Part model, mm, in its own coordinate system. A direction names the side the tool comes from. Round coordinates to 2 decimals unless told otherwise and drop trailing zeros. Write each loop counter-clockwise with the first axis right and the second up, starting at its lowest first coordinate (ties: lowest second). Pieces come first, ordered by that corner, then holes.
```python
from build123d import *

# Parameters (mm, degrees)
F0_W      = 25
F0_H      = 25
F1_DEPTH  = 30
F3_DEPTH  = 25.001
F4_R      = 2.1
F5_DEPTH  = 25.001
F6_R      = 5
F7_DEPTH  = 22
F9_DEPTH  = 7
F10_R     = 2.6
F11_DEPTH = 15
F14_W     = 30
F14_H     = 12.5
F15_DEPTH = 25
F16_DEPTH = 7
F18_DEPTH = 10
F20_DEPTH = 10
F22_D     = 8
F24_DEPTH = 12.5
F25_W     = 9.5
F25_H     = 25
F26_DEPTH = 3
F28_D     = 4.2
F28_DEPTH = 15
F28_TIP   = 1.2618073
F31_D     = 2.5
F31_DEPTH = 8
F31_TIP   = 0.7510757738


with BuildPart() as f1:
    # F0 (on Right) → F1 (new body, symmetric)
    with BuildSketch(Plane.YZ):
        Rectangle(F0_W, F0_H)
    extrude(amount=F1_DEPTH, both=True)

    # F2 (on face) → F3 (cut, through all)
    with BuildSketch(Plane.XY.offset(12.5)):
        with BuildLine():
            Line((12, -12.5), (22, -12.5))
            ThreePointArc((22, -12.5), (17, -7.5), (12, -12.5))
        make_face()
    extrude(amount=-F3_DEPTH, mode=Mode.SUBTRACT)

    # F4 (on face) → F5 (cut, through all)
    with BuildSketch(Plane.XY.offset(12.5)):
        with Locations((17, -4.5)):
            Circle(F4_R)
    extrude(amount=-F5_DEPTH, mode=Mode.SUBTRACT)

    # F6 (on face) → F7 (cut)
    with BuildSketch(Plane(origin=(0, 0, -12.5), x_dir=(1, 0, 0), z_dir=(0, 0, -1))):
        with Locations((5, 5.5)):
            Circle(F6_R)
    extrude(amount=-F7_DEPTH, mode=Mode.SUBTRACT)

    # F8 (on face) → F9 (cut)
    with BuildSketch(Plane.XZ.offset(12.5)):
        with BuildLine():
            Line((1.5, -12.5), (8.5, -12.5))
            Line((8.5, -12.5), (8.5, 2.5))
            ThreePointArc((8.5, 2.5), (5, 6), (1.5, 2.5))
            Line((1.5, 2.5), (1.5, -12.5))
        make_face()
    extrude(amount=-F9_DEPTH, mode=Mode.SUBTRACT)

    # F10 (on face) → F11 (cut)
    with BuildSketch(Plane(origin=(0, 0, -12.5), x_dir=(1, 0, 0), z_dir=(0, 0, -1))):
        with Locations((17, 4.5)):
            Circle(F10_R)
    extrude(amount=-F11_DEPTH, mode=Mode.SUBTRACT)


with BuildPart() as f12_1:
    # F12: copy of F1
    add(f1.part)


with BuildPart() as f1_1:
    add(f1.part)

    # F14 (on face) → F15 (join)
    with BuildSketch(Plane(origin=(0, 0, -12.5), x_dir=(1, 0, 0), z_dir=(0, 0, -1))):
        with Locations((15, -6.25)):
            Rectangle(F14_W, F14_H)
    extrude(amount=F15_DEPTH)

    # F16 (add): a face of the model
    f16_faces = [f1_1.faces().sort_by_distance(p)[0] for p in [
        (5, 12.5, -8.3333333333),
    ]]
    extrude(f16_faces, amount=F16_DEPTH)

    # F17 (on face) → F18 (cut)
    with BuildSketch(Plane(origin=(0, 19.5, 0), x_dir=(-1, 0, 0), z_dir=(0, 1, 0))):
        Polygon((-30, -5), (-6.4768494526, 0), (30, 0), (30, 12.5), (-30, 12.5), align=None)
    extrude(amount=-F18_DEPTH, mode=Mode.SUBTRACT)

    # F19 (on face) → F20 (cut)
    with BuildSketch(Plane(origin=(0, 19.5, 0), x_dir=(-1, 0, 0), z_dir=(0, 1, 0))):
        Polygon((30, -1.2575895653), (-12.3933431868, -1.2575895653), (-4.6897810382, -37.5), (0, -37.5), (0, -12.5), (30, -12.5), align=None)
        Polygon((-12.3933431868, 5.6717685307), (-12.3933431868, -1.2575895653), (-6.4768494526, 0), (30, 0), (30, 5.6717685307), align=None)
        Polygon((-6.4768494526, 0), (-12.3933431868, -1.2575895653), (30, -1.2575895653), (30, 0), align=None)
    extrude(amount=-F20_DEPTH, mode=Mode.SUBTRACT)

    # F22 (through all)
    with Locations(Plane(origin=(0.2799765277, 0, 1.317186002), x_dir=(0.9781476007, 0, -0.2079116908), z_dir=(0.2079116908, 0, 0.9781476007))):
        with Locations((27.3839864761, 14.5)):
            Hole(F22_D / 2)

    # F23 (on face) → F24 (cut)
    with BuildSketch(Plane.XY.offset(12.5)):
        Polygon((21.3397459622, 2.5), (30, -12.5), (30, 9.5), (17.2982940778, 9.5), align=None)
        Polygon((-30, 2.5), (21.3397459622, 2.5), (17.2982940778, 9.5), (-30, 9.5), align=None)
    extrude(amount=-F24_DEPTH, mode=Mode.SUBTRACT)

    # F25 (on face) → F26 (cut)
    with BuildSketch(Plane.YZ.offset(30)):
        with BuildLine():
            Line((-12.5, 0), (-12.5, -12.5))
            Line((-12.5, -12.5), (0, -12.5))
            Line((0, -12.5), (9.5, -12.5))
            Line((9.5, -12.5), (19.5, -12.5))
            Line((19.5, -12.5), (19.5, -5))
            Line((19.5, -5), (17.1457513111, -5))
            add(Edge.make_bspline(
                [(14.5, -9.8097343447), (16.011857892, -9.8097343447), (17.1457513111, -5)],
                knots=[3.1415926536, 3.1415926536, 3.1415926536, 3.8643269014, 3.8643269014, 3.8643269014], degree=2, weights=[1, 0.9354143467, 1]))
            add(Edge.make_bspline(
                [(11.8542486889, -5), (12.988142108, -9.8097343447), (14.5, -9.8097343447)],
                knots=[2.4188584058, 2.4188584058, 2.4188584058, 3.1415926536, 3.1415926536, 3.1415926536], degree=2, weights=[1, 0.9354143467, 1]))
            Line((11.8542486889, -5), (9.5, -5))
            Line((9.5, -5), (9.5, 0))
            Line((9.5, 0), (-12.5, 0))
        make_face()
        with BuildLine():
            Line((-12.5, 12.5), (-12.5, 0))
            Line((-12.5, 0), (9.5, 0))
            Line((9.5, 0), (9.5, -5))
            Line((9.5, -5), (11.8542486889, -5))
            add(Edge.make_bspline(
                [(11.8542486889, -5), (12.988142108, -9.8097343447), (14.5, -9.8097343447)],
                knots=[2.4188584058, 2.4188584058, 2.4188584058, 3.1415926536, 3.1415926536, 3.1415926536], degree=2, weights=[1, 0.9354143467, 1]))
            add(Edge.make_bspline(
                [(14.5, -9.8097343447), (16.011857892, -9.8097343447), (17.1457513111, -5)],
                knots=[3.1415926536, 3.1415926536, 3.1415926536, 3.8643269014, 3.8643269014, 3.8643269014], degree=2, weights=[1, 0.9354143467, 1]))
            Line((17.1457513111, -5), (19.5, -5))
            Line((19.5, -5), (19.5, 12.5))
            Line((19.5, 12.5), (-12.5, 12.5))
        make_face()
        with Locations((4.75, -25)):
            Rectangle(F25_W, F25_H)
    extrude(amount=-F26_DEPTH, mode=Mode.SUBTRACT)

    # F28
    with Locations(Plane(origin=(12.1133666591, 0, -2.5747755673), x_dir=(0, -1, 0), z_dir=(-0.9781476007, 0, 0.2079116908))):
        with Locations((-14.5, -7.7054747223), (-14.5, -17.7054747223), (-14.5, -27.7054747223)):
            Hole(F28_D / 2, depth=F28_DEPTH)
            with Locations((0, 0, -(F28_DEPTH + F28_TIP / 2))):  # 118° drill point
                Cone(0, F28_D / 2, F28_TIP, mode=Mode.SUBTRACT)

    # F31
    with Locations(Plane(origin=(17.0873412263, 9.8653810568, 0), x_dir=(-0.5, 0.8660254038, 0), z_dir=(0.8660254038, 0.5, 0))):
        with Locations((-12.397114317, 9.5)):
            Hole(F31_D / 2, depth=F31_DEPTH)
            with Locations((0, 0, -(F31_DEPTH + F31_TIP / 2))):  # 118° drill point
                Cone(0, F31_D / 2, F31_TIP, mode=Mode.SUBTRACT)


solid = f1_1.part
```
Q1. Cut at B-B on y = -5.5. Write the cut outline in (x, z).
Values follow:
outline: (-30, -12.5) - (0, -12.5) - (0, 9.5) - (10, 9.5) - (10, -12.5) - (14.6, -12.5) - (14.6, 2.5) - (15.15, 2.5) - (15.15, 12.5) - (-30, 12.5) - close; (18.85, 2.5) - (19.4, 2.5) - (19.4, -12.5) - (27, -12.5) - (27, 0) - (25.96, 0) - (25.96, 12.5) - (18.85, 12.5) - close
Q2. Cut at C-C on x = -21. Write the cut outline in (y, z).
Values follow:
outline: (-12.5, -12.5) - (9.5, -12.5) - (9.5, 0) - (2.5, 0) - (2.5, 12.5) - (-12.5, 12.5) - close
Q3. Which spindle directions (+Z, -Z, +X, -X, +Y, -Y) get a long thin tool onto all of the face, cutting with end or side? Do faces 4 (the flat face through (24.13, -2.33, 6.34)), 5 (the cylindrical face through (15.334, -5.778, 7.57)), 6 (the flat face through (29.5, 13.3, -12.5)), 7 (the flat face through (-9, -12.5, 0)), 8 (the cylindrical face through (19.48, -5.28, -5.11)). Say none if no direction does.
Values follow:
face 4: +Z, +X, +Y
face 5: +Z, -Z
face 6: +Z, +X, +Y, -Y
face 7: +Z, -Z, +X, -X, -Y
face 8: -Z
Q4. Mould opens along Z. For faces 1 (the flat face through (27, 19, -8)), 2 (the cylindrical face through (5, -11, 6)), 3 (the cylindrical face through (12.235, 16.503, -30.28)) say: +Z half, -Z half, draft (parallel to the pull), parting line (faces both ways), or undercut.
Values follow:
face 1: draft
face 2: -Z half
face 3: undercut
Q5. Wall check: L1, parallel to Y at x = 17, z = 8; L2, parallel to X at y = -5.5, z = -3; L3, parallel to Z at x = 9, y = 8. Give the ranges that are in metal, low to high.
Values follow:
L1: y = -7.5 to -6.6, -2.4 to 2.5
L2: x = -30 to 0, 10 to 14.6, 19.4 to 27
L3: z = -37.5 to 0
Q6. Cut at A-A on z = 1.5. Write the cut outline in (x, y), plus the area to 3 significant figures.
Values follow:
outline: (-30, -12.5) - (1.5, -12.5) - (1.5, -9.07) arc R5 cw (long way) to (8.5, -9.07) - (8.5, -12.5) - (12, -12.5) arc R5 cw to (22, -12.5) - (27, -12.5) - (27, -7.3) - (21.34, 2.5) - (-30, 2.5) - close; hole circle Ø5.2 at (17, -4.5)
area: 671 mm2
Q7. Drop flat-ended pins along their axis: pin 1 (8 mm diameter, centred on x = -7.5, y = -6.5, fed in from -Z); pin 2 (19 mm diameter, centred on x = -11.5, z = -18.5, fed in from +Y); pin 3 (5 mm diameter, centred on y = 7, z = -29, fed in from -X). Give the stop position or say it passes through.
Values follow:
pin 1: stops at z = -12.5
pin 2: stops at y = 9.5
pin 3: stops at x = 0
